Part print with two shaded views. Sizes in mm from the minimum x, y, z corner. A direction names the side the tool comes from. Round coordinates to 2 decimals unless told otherwise and drop trailing zeros. Loops run counter-clockwise (first coordinate to the right, second up) from the corner with the lowest first, then second, coordinate; pieces in that order, holes last.
(1) Cut at B-B on z = 1.5. List the corners of the cut face in (x, y) (1 decimal), then the cut area to 3 significant figures.
(2) Cut at A-A on y = 13.7. List the corners of the cut face in (x, z) (1 decimal), then the cut area to 3 significant figures.
(3) Cut at C-C on x = 6. List the corners of the cut face in (y, z), then the cut area to 3 significant figures.
(4) Mould opens along Y. For the marked faces 3, 4 and 5 say: +Y half, -Y half, draft (parallel to the pull), parting line (faces both ways), or undercut.
(5) Probe probe 1 along Y at (x, z) = (18, 10.25); probe 2 along Y at (x, z) = (6, 14.25); probe 3 along X at (y, z) = (16.05, 7.5) (1 decimal). List the from-to ranges inside material, lowest first.
(6) Cut at D-D on z = 7.5. List the corners of the cut face in (x, y) (1 decimal), then the cut area to 3 significant figures.
(7) Tool access for the marked faces 1 and 2: list every direction of +Z, -Z, +X, -X, +Y, -Y with a clear straight run to the whole face (end or side of a thin tool).
(8) Flat gauge pins, fed straight in: pin 1 (1 mm diameter, centred on y = 8, z = 6, fed in from +X); pin 2 (4 mm diameter, centred on x = 17, z = 5, fed in from +Y); pin 3 (4 mm diameter, centred on y = 19, z = 11.5, fed in from -X). Where does each tip first touch, or does it go through?
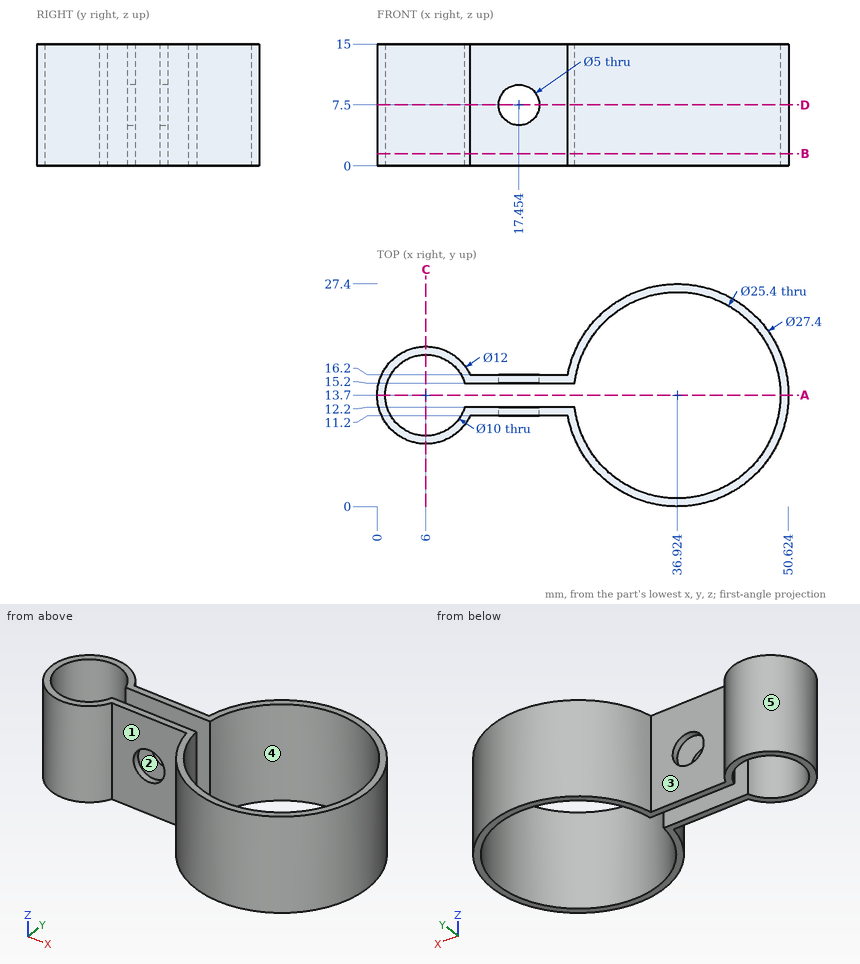
Final values:
1. outline: (11.5, 11.2) - (23.5, 11.2) arc R13.7 ccw (long way) to (23.5, 16.2) - (11.5, 16.2) arc R6 ccw (long way) to start; hole (10.8, 12.2) - (24.3, 12.2) arc R12.7 ccw (long way) to (24.3, 15.2) - (10.8, 15.2) arc R5 ccw (long way) to start
1. area: 135 mm2
2. outline: (0, 0) - (1, 0) - (1, 15) - (0, 15) - close; (49.6, 0) - (50.6, 0) - (50.6, 15) - (49.6, 15) - close
2. area: 30.0 mm2
3. outline: (7.7, 0) - (8.7, 0) - (8.7, 15) - (7.7, 15) - close; (18.7, 0) - (19.7, 0) - (19.7, 15) - (18.7, 15) - close
3. area: 30.0 mm2
4. face 3: +Y half
4. face 4: undercut
4. face 5: parting line
5. probe 1: y = 11.2 to 12.2, 15.2 to 16.2
5. probe 2: y = 7.7 to 8.7, 18.7 to 19.7
5. probe 3: x = 0.5 to 1.6, 10.4 to 15, 20 to 24.4, 49.4 to 50.4
6. outline: (10.8, 12.2) arc R5 cw (long way) to (10.8, 15.2) - (15, 15.2) - (15, 16.2) - (11.5, 16.2) arc R6 ccw (long way) to (11.5, 11.2) - (15, 11.2) - (15, 12.2) - close; (20, 11.2) - (23.5, 11.2) arc R13.7 ccw (long way) to (23.5, 16.2) - (20, 16.2) - (20, 15.2) - (24.3, 15.2) arc R12.7 cw (long way) to (24.3, 12.2) - (20, 12.2) - close
6. area: 125 mm2
7. face 1: +Z, -Z, -Y
7. face 2: +Z, -Z
8. pin 1: stops at x = 49.6
8. pin 2: stops at y = 16.2
8. pin 3: stops at x = 0.99
